For this review, take the finished solid that the model builds, in its own axes (mm). Face numbers are marked on the shaded views. Give positions to 0.01 mm unless a question says otherwise; leave off trailing zeros. Order: outer loops, then holes, each group sorted by start corner. A loop starts at its lowest first (then second) coordinate and runs counter-clockwise, first axis right, second up. Notation, with made-up numbers: (-36, -5) - (22, -5) arc R19 ccw to (22, 30) - close; hole circle Ø5 at (37.5, 30.25). An arc over 180 degrees is marked (long way). One line per item, written item: value.
```python
from build123d import *

# Parameters (mm, degrees)
F0_W     = 142.5278559327
F0_H     = 162.6823693514
F1_DEPTH = 100
F3_D     = 50
F5_D     = 50
F7_W     = 217.2406986356
F7_H     = 260.2855265141
F8_DEPTH = 100


with BuildPart() as f1:
    # F0 (on Top) → F1 (new body)
    with BuildSketch(Plane.XY):
        with Locations((3.5334713757, 13.1870955229)):
            Rectangle(F0_W, F0_H)
    extrude(amount=F1_DEPTH)

    # F3 (through all)
    with Locations(Plane.XY.offset(100)):
        with Locations((0, 18.059482798)):
            Hole(F3_D / 2)

    # F5 (through all)
    with Locations(Plane.YZ.offset(74.7973993421)):
        with Locations((0, 49.8763620853)):
            Hole(F5_D / 2)

    # F7 (on 3pt) → F8 (cut)
    with BuildSketch(Plane(origin=(-33.5460278912, -29.390052834, 47.8124343039), x_dir=(0.8583543186, -0.2686733101, 0.4370841066), z_dir=(-0.5130573689, -0.449495339, 0.7312496676))):
        with Locations((4.2272098362, 30.3416997194)):
            Rectangle(F7_W, F7_H)
    extrude(amount=F8_DEPTH, mode=Mode.SUBTRACT)


solid = f1.part
```
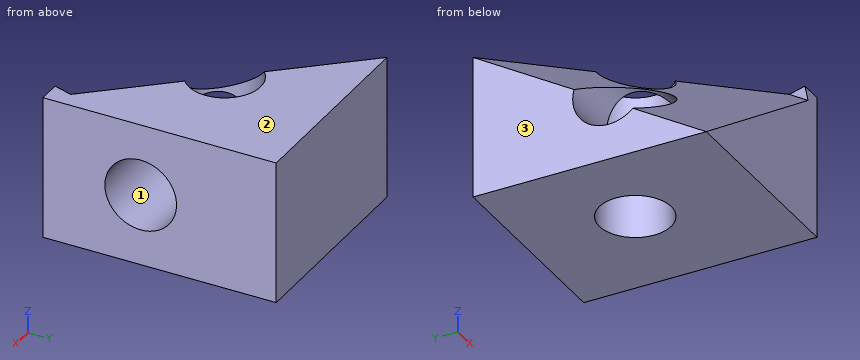
(1) Take a section at C-C (z = 42). Write out the cut boundary in (x, y).
Answers below:
outline: (-67.73, 23.73) - (-24.35, 23.73) arc R25 cw to (24.35, 23.73) - (74.8, 23.73) - (74.8, 94.53) - (-67.73, 94.53) - close; (-46.79, -23.73) - (-7.87, -68.15) - (74.8, -68.15) - (74.8, -23.73) - close
(2) For P1, Ø4, axis at y = 39.5, z = 78, coming from the -X side, flat-tipped, find the tip position at first contact; note if it passes through.
Answers below:
P1: stops at x = -54.22
(3) Take a section at A-A (y = 41). Write out the cut boundary in (x, z).
Answers below:
outline: (-67.73, 0) - (-9.94, 0) - (-9.94, 100) - (-20.83, 100) - (-67.73, 67.1) - close; (9.94, 0) - (74.8, 0) - (74.8, 100) - (9.94, 100) - close
(4) Take a section at B-B (x = 0). Write out the cut boundary in (y, z), then the cut area to 3 significant figures.
Answers below:
outline: (-68.15, 0) - (-6.94, 0) - (-6.94, 25.86) arc R25 cw to (-6.94, 73.89) - (-6.94, 85.15) - (-68.15, 47.52) - close; (43.06, 0) - (94.53, 0) - (94.53, 100) - (43.06, 100) - close
area: 8,570 mm^2
(5) Take a section at D-D (x = -46.5). Write out the cut boundary in (y, z).
Answers below:
outline: (-68.15, 0) - (94.53, 0) - (94.53, 100) - (70.3, 100) - (17.61, 67.62) arc R25 cw (long way) to (-23.78, 42.17) - (-68.15, 14.9) - close
(6) Wall thickness on line 1 (X direction, y = 18, z = 20.5); line 2 (Z direction, x = 19, y = 1); line 3 (Y direction, x = -9.5, z = 47): over which ranges is each line inside the solid? List them lowest first. Write a range as from..to.
Answers below:
line 1: x = -67.73..-25, 25..74.8
line 2: z = 0..24.9, 74.86..100
line 3: y = -58.16..-24.83, 41.18..94.53
(7) Draft analysis for pull direction Z (two halves, no side actions). For the marked faces 1, 2 and 3, state which applies: pulls with the +Z half, pulls with the -Z half, needs draft (parallel to the pull), parting line crosses it, or undercut.
Answers below:
face 1: undercut
face 2: pulls with the +Z half
face 3: needs draft
